Job drawing, mm, ordinate dimensions from the low corner. One solid piece. A direction names the side the tool comes from. Give positions to 0.01 mm unless a question says otherwise; leave off trailing zeros. Order: outer loops, then holes, each group sorted by start corner. A loop starts at its lowest first (then second) coordinate and runs counter-clockwise, first axis right, second up.
Item 1: Band-saw the part on B-B on y = 9. Give the cut face in (x, z), plus the area to 3 significant figures.
Item 2: Band-saw the part on D-D on x = 6.75. Give the cut face in (y, z) (1 decimal), plus the area to 3 significant figures.
Item 3: Band-saw the part on A-A on x = 9.6. Give the cut face in (y, z).
Item 4: Band-saw the part on C-C on z = 0.75. Give the cut face in (x, y), plus the area to 3 significant figures.
Item 5: Which spindle directions (+Z, -Z, +X, -X, +Y, -Y) get a long thin tool onto all of the face, cutting with end or side? Do the marked faces 4, 5 and 6. Say none if no direction does.
Item 6: Two-plate mould, pull along Y, no slides. Class the marked faces 1, 2 and 3: released by +Y, released by -Y, zero draft, split by the parting line, or undercut.
Item 7: Flat gauge pins, fed straight in: P1, Ø1.5, axis at y = 22, z = 0.5, coming from the +X side; P2, Ø2, axis at x = 1, z = 1.5, coming from the -Y side. Where does each tip first touch, or does it go through?
Item 8: Wall check: L1, parallel to Y at x = 9.6, z = 2.2; L2, parallel to X at y = 10.5, z = 1.75; L3, parallel to Y at x = 10.25, z = 3.7. Give the ranges that are in metal, low to high.
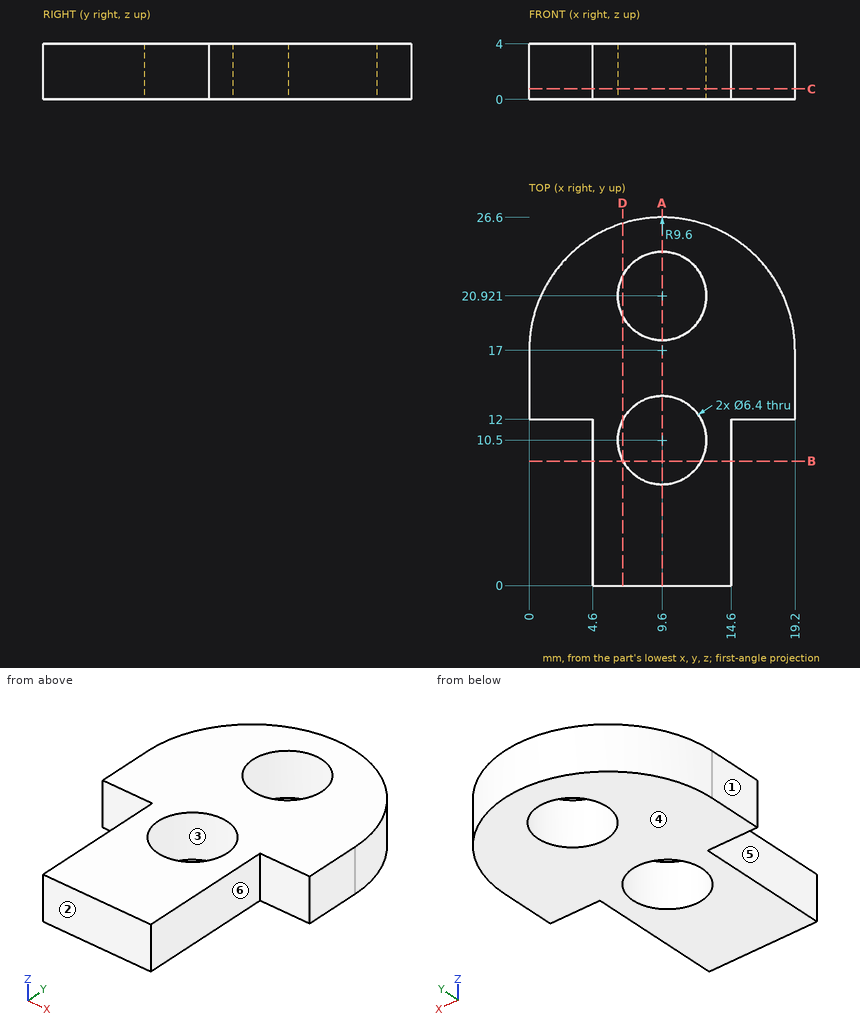
The answers:
1. outline: (4.6, 0) - (6.77, 0) - (6.77, 4) - (4.6, 4) - close; (12.43, 0) - (14.6, 0) - (14.6, 4) - (12.43, 4) - close
1. area: 17.4 mm2
2. outline: (0, 0) - (9, 0) - (9, 4) - (0, 4) - close; (12, 0) - (19.5, 0) - (19.5, 4) - (12, 4) - close; (22.4, 0) - (26.2, 0) - (26.2, 4) - (22.4, 4) - close
2. area: 81.4 mm2
3. outline: (0, 0) - (7.3, 0) - (7.3, 4) - (0, 4) - close; (13.7, 0) - (17.72, 0) - (17.72, 4) - (13.7, 4) - close; (24.12, 0) - (26.6, 0) - (26.6, 4) - (24.12, 4) - close
4. outline: (0, 12) - (4.6, 12) - (4.6, 0) - (14.6, 0) - (14.6, 12) - (19.2, 12) - (19.2, 17) arc R9.6 ccw to (0, 17) - close; hole circle Ø6.4 at (9.6, 10.5); hole circle Ø6.4 at (9.6, 20.92)
4. area: 296 mm2
5. face 4: -Z, +X, -X, +Y, -Y
5. face 5: +Z, -Z, -X, -Y
5. face 6: +Z, -Z, +X, -Y
6. face 1: zero draft
6. face 2: released by -Y
6. face 3: undercut
7. P1: stops at x = 18.21
7. P2: stops at y = 12
8. L1: y = 0 to 7.3, 13.7 to 17.72, 24.12 to 26.6
8. L2: x = 4.6 to 6.4, 12.8 to 14.6
8. L3: y = 0 to 7.37, 13.63 to 17.79, 24.05 to 26.58
